```python
from build123d import *

# Parameters (mm, degrees)
SKETCH1_W                = 130.175
SKETCH1_H                = 130.175
BOSS_EXTRUDE1_DEPTH      = 19.05
CUT_EXTRUDE1_REACH       = 21.05
SKETCH2_R                = 7.9375
SKETCH3_R                = 12.7
BOSS_EXTRUDE2_DEPTH      = 33.3375
CUT_EXTRUDE2_REACH       = 98.837
SKETCH4_W                = 28.575
SKETCH4_H                = 82.55
SKETCH5_R                = 57.15
SKETCH5_R_2              = 50.8
BOSS_EXTRUDE3_DEPTH      = 666.75
FILLET1_R                = 9.525
SKETCH6_R                = 7.9375
BOSS_EXTRUDE4_DEPTH      = 19.05
CUT_EXTRUDE3_REACH       = 808.45
SKETCH7_R                = 25.4
SKETCH8_R                = 7.9375
BOSS_EXTRUDE5_DEPTH      = 19.05
BOSS_EXTRUDE5_DEPTH_BACK = 730.25


with BuildPart() as part:
    # Sketch1 → Boss-Extrude1 (new body)
    with BuildSketch(Plane(origin=(0, 0, 0), x_dir=(1, 0, 0), z_dir=(0, 1, 0))):
        Rectangle(SKETCH1_W, SKETCH1_H)
    extrude(amount=BOSS_EXTRUDE1_DEPTH)

    # Sketch2 → Cut-Extrude1 (cut, up to next)
    with BuildSketch(Plane(origin=(0, 19.05, 0), x_dir=(1, 0, 0), z_dir=(0, 1, 0)), mode=Mode.PRIVATE) as cut_extrude1_sk1:
        with Locations(Location((-50.8, 50.8, 0), (0, 0, 270))):  # turned: the seam where the file's is
            Circle(SKETCH2_R)
    cut_extrude1_tool1 = extrude(cut_extrude1_sk1.sketch, amount=-CUT_EXTRUDE1_REACH, mode=Mode.PRIVATE) & part.part
    add(cut_extrude1_tool1.solids().sort_by_distance((-50.8, 19.05, -50.8))[0], mode=Mode.SUBTRACT)
    # Sketch2 → Cut-Extrude1 (cut, up to next)
    with BuildSketch(Plane(origin=(0, 19.05, 0), x_dir=(1, 0, 0), z_dir=(0, 1, 0)), mode=Mode.PRIVATE) as cut_extrude1_sk2:
        with Locations(Location((50.8, 50.8, 0), (0, 0, 270))):  # turned: the seam where the file's is
            Circle(SKETCH2_R)
    cut_extrude1_tool2 = extrude(cut_extrude1_sk2.sketch, amount=-CUT_EXTRUDE1_REACH, mode=Mode.PRIVATE) & part.part
    add(cut_extrude1_tool2.solids().sort_by_distance((50.8, 19.05, -50.8))[0], mode=Mode.SUBTRACT)
    # Sketch2 → Cut-Extrude1 (cut, up to next)
    with BuildSketch(Plane(origin=(0, 19.05, 0), x_dir=(1, 0, 0), z_dir=(0, 1, 0)), mode=Mode.PRIVATE) as cut_extrude1_sk3:
        with Locations(Location((50.8, -50.8, 0), (0, 0, 270))):  # turned: the seam where the file's is
            Circle(SKETCH2_R)
    cut_extrude1_tool3 = extrude(cut_extrude1_sk3.sketch, amount=-CUT_EXTRUDE1_REACH, mode=Mode.PRIVATE) & part.part
    add(cut_extrude1_tool3.solids().sort_by_distance((50.8, 19.05, 50.8))[0], mode=Mode.SUBTRACT)
    # Sketch2 → Cut-Extrude1 (cut, up to next)
    with BuildSketch(Plane(origin=(0, 19.05, 0), x_dir=(1, 0, 0), z_dir=(0, 1, 0)), mode=Mode.PRIVATE) as cut_extrude1_sk4:
        with Locations(Location((-50.8, -50.8, 0), (0, 0, 270))):  # turned: the seam where the file's is
            Circle(SKETCH2_R)
    cut_extrude1_tool4 = extrude(cut_extrude1_sk4.sketch, amount=-CUT_EXTRUDE1_REACH, mode=Mode.PRIVATE) & part.part
    add(cut_extrude1_tool4.solids().sort_by_distance((-50.8, 19.05, 50.8))[0], mode=Mode.SUBTRACT)

    # Sketch3 → Boss-Extrude2 (add, symmetric)
    with BuildSketch(Plane(origin=(0, 0, 0), x_dir=(0, 0, -1), z_dir=(1, 0, 0))):
        with BuildLine():
            Line((-31.75, 19.05), (-31.75, 88.9))
            ThreePointArc((-31.75, 88.9), (0, 120.65), (31.75, 88.9))
            Line((31.75, 88.9), (31.75, 19.05))
            Line((31.75, 19.05), (-31.75, 19.05))
        make_face()
        with Locations((0, 88.9)):
            Circle(SKETCH3_R, mode=Mode.SUBTRACT)
    extrude(amount=BOSS_EXTRUDE2_DEPTH, both=True)

    # Sketch4 → Cut-Extrude2 (cut, up to next)
    with BuildSketch(Plane.XY.offset(31.75), mode=Mode.PRIVATE) as cut_extrude2_sk1:
        with Locations((0, 79.375)):
            Rectangle(SKETCH4_W, SKETCH4_H)
    cut_extrude2_tool1 = extrude(cut_extrude2_sk1.sketch, amount=-CUT_EXTRUDE2_REACH, mode=Mode.PRIVATE) & part.part
    add(cut_extrude2_tool1.solids().sort_by_distance((0, 79.375, 31.75))[0], mode=Mode.SUBTRACT)

    # Sketch5 → Boss-Extrude3 (add)
    with BuildSketch(Plane.XZ):
        with Locations(Location((0, 0, 0), (0, 0, 90))):  # turned: the seam where the file's is
            Circle(SKETCH5_R)
        with Locations(Location((0, 0, 0), (0, 0, 270))):  # turned: the seam where the file's is
            Circle(SKETCH5_R_2, mode=Mode.SUBTRACT)
    extrude(amount=BOSS_EXTRUDE3_DEPTH)

    # Fillet1
    fillet1_edges = [part.edges().sort_by_distance(p)[0] for p in [
        (65.0875, 9.525, 65.0875),
        (-65.0875, 9.525, 65.0875),
        (-65.0875, 9.525, -65.0875),
        (65.0875, 9.525, -65.0875),
    ]]
    fillet(fillet1_edges, radius=FILLET1_R)

    # Sketch6 → Boss-Extrude4 (add)
    with BuildSketch(Plane.XZ.offset(666.75)):
        with BuildLine():
            Line((-65.0875, 55.5625), (-65.0875, -55.5625))
            ThreePointArc((-65.0875, -55.5625), (-62.297692091, -62.297692091), (-55.5625, -65.0875))
            Line((-55.5625, -65.0875), (55.5625, -65.0875))
            ThreePointArc((55.5625, -65.0875), (62.297692091, -62.297692091), (65.0875, -55.5625))
            Line((65.0875, -55.5625), (65.0875, 55.5625))
            ThreePointArc((65.0875, 55.5625), (62.297692091, 62.297692091), (55.5625, 65.0875))
            Line((55.5625, 65.0875), (-55.5625, 65.0875))
            ThreePointArc((-55.5625, 65.0875), (-62.297692091, 62.297692091), (-65.0875, 55.5625))
        make_face()
        with Locations(Location((-50.8, 50.8, 0), (0, 0, 90))):  # turned: the seam where the file's is
            Circle(SKETCH6_R, mode=Mode.SUBTRACT)
        with Locations(Location((50.8, 50.8, 0), (0, 0, 90))):  # turned: the seam where the file's is
            Circle(SKETCH6_R, mode=Mode.SUBTRACT)
        with Locations(Location((50.8, -50.8, 0), (0, 0, 90))):  # turned: the seam where the file's is
            Circle(SKETCH6_R, mode=Mode.SUBTRACT)
        with Locations(Location((-50.8, -50.8, 0), (0, 0, 90))):  # turned: the seam where the file's is
            Circle(SKETCH6_R, mode=Mode.SUBTRACT)
    extrude(amount=BOSS_EXTRUDE4_DEPTH)

    # Sketch7 → Cut-Extrude3 (cut, up to next)
    with BuildSketch(Plane.XZ.offset(685.8), mode=Mode.PRIVATE) as cut_extrude3_sk1:
        with Locations(Location((0, 0, 0), (0, 0, 270))):  # turned: the seam where the file's is
            Circle(SKETCH7_R)
    cut_extrude3_tool1 = extrude(cut_extrude3_sk1.sketch, amount=-CUT_EXTRUDE3_REACH, mode=Mode.PRIVATE) & part.part
    add(cut_extrude3_tool1.solids().sort_by_distance((0, -685.8, 0))[0], mode=Mode.SUBTRACT)

    # Sketch8 → Boss-Extrude5 (add, two sides)
    with BuildSketch(Plane(origin=(0, 19.05, 0), x_dir=(1, 0, 0), z_dir=(0, 1, 0))) as boss_extrude5_sk:
        with Locations(Location((-50.8, 50.8, 0), (0, 0, 270))):  # turned: the seam where the file's is
            Circle(SKETCH8_R)
        with Locations(Location((50.8, 50.8, 0), (0, 0, 270))):  # turned: the seam where the file's is
            Circle(SKETCH8_R)
        with Locations(Location((50.8, -50.8, 0), (0, 0, 270))):  # turned: the seam where the file's is
            Circle(SKETCH8_R)
        with Locations(Location((-50.8, -50.8, 0), (0, 0, 270))):  # turned: the seam where the file's is
            Circle(SKETCH8_R)
    extrude(amount=BOSS_EXTRUDE5_DEPTH)
    extrude(boss_extrude5_sk.sketch, amount=-BOSS_EXTRUDE5_DEPTH_BACK)


solid = part.part
```
The listing builds one solid part. Answer for the finished solid, in the listing's coordinates (mm). A direction names the side the tool comes from. Coordinates: 2 decimals unless noted, no trailing zeros. Loops run counter-clockwise (first coordinate to the right, second up) from the corner with the lowest first, then second, coordinate; pieces in that order, holes last. Notation, with made-up numbers: M 5.25,38 L 29.25,38 A20 ccw 29.25,77 Z; hole C -21,-4 d5. An arc over 180 degrees is marked long. Answer as CSV lines item,"result". Start each with the question number.
(1) The part is cut by section A-A (y = -423.5). State how many separate pieces and enclosed holes the cut face has, and give its area (3 significant figures).
(2) The mould has two halves that part along Z. Classify faces 6 (the flat face through (15, 54, -31.75)), 7 (the cylindrical face through (56.165, 28.442, 44.95)), 8 (the flat face through (51, -711.2, -51)), 9 (the flat face through (-1, 19.05, -44)): pulls with the +Z half, pulls with the -Z half, needs draft (parallel to the pull), parting line crosses it, or undercut.
(3) Given pin 1 (6 mm diameter, centred on x = 30.5, z = 30, fed in from -Y); pin 2 (2 mm diameter, centred on y = -563.5, z = -44.5, fed in from -X); pin 3 (10 mm diameter, centred on y = 31, z = -48, fed in from -X), each flat-ended and moving along its own axis, determine where each tip first touches the part or whether it passes through.
(4) For faces 1 (the flat face through (-33.338, 71, 0)), 2 (the cylindrical face through (-55.63, -698.32, -57.1)), 3 (the flat face through (14.288, 70, 0)), 4 (the cylindrical face through (56.165, -328.708, 44.95)), 5 (the cylindrical face through (-55.63, 28.44, 44.5)), determine the directions among +Z, -Z, +X, -X, +Y, -Y from which every point of the face is accessible in a straight line to the end or side of a thin tool.
(5) Find the intervals of material crossed by L1, parallel to Y at x = 28, z = 0; L2, parallel to Y at x = -25, z = 0; L3, parallel to Y at x = -59, z = 7, in increasing order. Write a range as [from, to].
(6) The part is cut by section B-B (x = 0). Give the vertices of the cut face in (y, z), and give its area (3 significant figures).
Determined:
1,separate pieces,"5"
1,enclosed holes,"1"
1,area,"2,950 mm2"
2,face 6,"pulls with the -Z half"
2,face 7,"undercut"
2,face 8,"needs draft"
2,face 9,"undercut"
3,pin 1,"y = -685.8"
3,pin 2,"x = -56.71"
3,pin 3,"x = -58.74"
4,face 1,"+Z, -Z, -X, +Y"
4,face 2,"-Y"
4,face 3,"+Z, -Z, +Y"
4,face 4,"none"
4,face 5,"+Y"
5,L1,"[-685.8, -666.75], [0, 76.2], [101.6, 120.65]"
5,L2,"[0, 76.2], [101.6, 120.65]"
5,L3,"[-685.8, -666.75], [0, 19.05]"
6,outline,"M -685.8,-65.09 L -666.75,-65.09 L -666.75,-57.15 L 0,-57.15 L 0,-65.09 L 19.05,-65.09 L 19.05,-31.75 L 38.1,-31.75 L 38.1,31.75 L 19.05,31.75 L 19.05,65.09 L 0,65.09 L 0,57.15 L -666.75,57.15 L -666.75,65.09 L -685.8,65.09 L -685.8,25.4 L -666.75,25.4 L -666.75,50.8 L 0,50.8 L 0,-50.8 L -666.75,-50.8 L -666.75,-25.4 L -685.8,-25.4 Z"
6,area,"13,700 mm2"
